The model under review builds one solid part; all positions refer to its coordinate system, in mm. A direction names the side the tool comes from. Round coordinates to 2 decimals unless told otherwise and drop trailing zeros. Order: outer loops, then holes, each group sorted by start corner. A loop starts at its lowest first (then second) coordinate and runs counter-clockwise, first axis right, second up.
1) Consider section C-C (z = 16.5). Give the boundary of the cut face in (x, y), then the cut area to 3 significant figures.
2) To check wall thickness, follow L1, parallel to X at y = 15, z = 0; L2, parallel to Z at x = 26, y = 6; L3, parallel to X at y = 9.5, z = 0. State the ranges of each line that lie inside material, in increasing order.
3) Machinability: for faces 4 (the face through (51.505, 24.79, 19.295)), 5 (the face through (-40, 20, 0)), 6 (the face through (85, 10, 0)), which of the approach directions +Z, -Z, +X, -X, +Y, -Y give a long, thin tool a straight path to every point of the face, cutting with its end or side? Answer none if there is none.
4) Consider section A-A (z = 0). Give the boundary of the cut face in (x, y).
5) Consider section D-D (y = 34). Give the boundary of the cut face in (x, z), then the cut area to 3 significant figures.
6) Clearance check with flat-ended pins moving along their axes: P1, Ø1.5, axis at y = 11.5, z = 21.5, coming from the -X side; P2, Ø2, axis at y = 16.5, z = 11.5, coming from the -X side; P3, Ø10.5, axis at x = 63.5, y = 21.5, coming from the -Z side. State where each tip first meets the part, or that it passes through.
7) Consider section B-B (y = 4). Give the boundary of the cut face in (x, z), then the cut area to 3 significant figures.
8) Mouldability with a two-part tool opening along Z and no side actions: class faces 1 (the face through (-77.93, 19.72, 0.65)), 2 (the face through (-65, 25, -8)), 3 (the face through (-97.15, 4.93, 26.99)) as pulls with the +Z half, pulls with the -Z half, needs draft (parallel to the pull), parting line crosses it, or undercut.
from build123d import *

# Parameters (mm, degrees)
EXTRUDE_2_DEPTH     = 10
EXTRUDE_3_DEPTH     = 30
SKETCH_7_R          = 3
CUT_EXTRUDE_3_DEPTH = 40


with BuildPart() as part:
    # 草图1 → 凸台-拉伸2 (new body)
    with BuildSketch(Plane(origin=(0, 0, 0), x_dir=(1, 0, 0), z_dir=(0, 1, 0))):
        with BuildLine():
            Line((100, -20), (100, 20))
            ThreePointArc((100, 20), (97.071067812, 27.071067812), (90, 30))
            Line((90, 30), (-90, 30))
            ThreePointArc((-90, 30), (-97.071067812, 27.071067812), (-100, 20))
            Line((-100, 20), (-100, -20))
            ThreePointArc((-100, -20), (-97.071067812, -27.071067812), (-90, -30))
            Line((-90, -30), (90, -30))
            ThreePointArc((90, -30), (97.071067812, -27.071067812), (100, -20))
        make_face()
    extrude(amount=EXTRUDE_2_DEPTH)

    # 草图5 → 凸台-拉伸3 (add)
    with BuildSketch(Plane(origin=(0, 10, 0), x_dir=(1, 0, 0), z_dir=(0, 1, 0))):
        with BuildLine():
            Line((-46.097722286, 30), (46.097722286, 30))
            ThreePointArc((46.097722286, 30), (51.446141019, 19.449796252), (54.415071442, 8))
            Line((54.415071442, 8), (75, 8))
            ThreePointArc((75, 8), (83, 0), (75, -8))
            Line((75, -8), (54.415071442, -8))
            ThreePointArc((54.415071442, -8), (51.446141019, -19.449796252), (46.097722286, -30))
            Line((46.097722286, -30), (-46.097722286, -30))
            ThreePointArc((-46.097722286, -30), (-51.446141019, -19.449796252), (-54.415071442, -8))
            Line((-54.415071442, -8), (-75, -8))
            ThreePointArc((-75, -8), (-83, 0), (-75, 8))
            Line((-75, 8), (-54.415071442, 8))
            ThreePointArc((-54.415071442, 8), (-51.446141019, 19.449796252), (-46.097722286, 30))
        make_face()
    extrude(amount=EXTRUDE_3_DEPTH)

    # 草图7 → 切除-拉伸3 (cut)
    with BuildSketch(Plane.XZ):
        with Locations(Location((-75, 0, 0), (0, 0, 270))):
            Circle(SKETCH_7_R)
        with Locations(Location((75, 0, 0), (0, 0, 90))):
            Circle(SKETCH_7_R)
        with BuildLine():
            Line((34.641016151, -20), (-34.641016151, -20))
            ThreePointArc((-34.641016151, -20), (-40, 0), (-34.641016151, 20))
            Line((-34.641016151, 20), (34.641016151, 20))
            ThreePointArc((34.641016151, 20), (40, 0), (34.641016151, -20))
        make_face()
    extrude(amount=-CUT_EXTRUDE_3_DEPTH, mode=Mode.SUBTRACT)


solid = part.part
Answer below:
1. outline: (-100, 0) - (-36.44, 0) - (-36.44, 40) - (-52.47, 40) - (-52.47, 10) - (-100, 10) - close; (36.44, 0) - (100, 0) - (100, 10) - (52.47, 10) - (52.47, 40) - (36.44, 40) - close
1. area: 2,230 mm2
2. L1: x = -83 to -78, -72 to -40, 40 to 72, 78 to 83
2. L2: z = -30 to -20, 20 to 30
2. L3: x = -100 to -78, -72 to -40, 40 to 72, 78 to 100
3. face 4: +Z, +X, +Y
3. face 5: +Y, -Y
3. face 6: +X, +Y
4. outline: (-100, 0) - (-78, 0) - (-78, 40) - (-83, 40) - (-83, 10) - (-100, 10) - close; (-72, 0) - (-40, 0) - (-40, 40) - (-72, 40) - close; (40, 0) - (72, 0) - (72, 40) - (40, 40) - close; (78, 0) - (100, 0) - (100, 10) - (83, 10) - (83, 40) - (78, 40) - close
5. outline: (-75, -8) - (-54.42, -8) arc R55 ccw to (-46.1, -30) - (46.1, -30) arc R55 ccw to (54.42, -8) - (75, -8) arc R8 ccw to (75, 8) - (54.42, 8) arc R55 ccw to (46.1, 30) - (-46.1, 30) arc R55 ccw to (-54.42, 8) - (-75, 8) arc R8 ccw to start; hole circle Ø6 at (-75, 0); hole (-34.64, -20) - (34.64, -20) arc R40 ccw to (34.64, 20) - (-34.64, 20) arc R40 ccw to start; hole circle Ø6 at (75, 0)
5. area: 3,990 mm2
6. P1: stops at x = -50.94
6. P2: stops at x = -53.99
6. P3: stops at z = -8
7. outline: (-100, -20) arc R10 ccw to (-90, -30) - (90, -30) arc R10 ccw to (100, -20) - (100, 20) arc R10 ccw to (90, 30) - (-90, 30) arc R10 ccw to (-100, 20) - close; hole circle Ø6 at (-75, 0); hole (-34.64, -20) - (34.64, -20) arc R40 ccw to (34.64, 20) - (-34.64, 20) arc R40 ccw to start; hole circle Ø6 at (75, 0)
7. area: 8,800 mm2
8. face 1: undercut
8. face 2: pulls with the -Z half
8. face 3: pulls with the +Z half
